```python
from build123d import *

# Parameters (mm, degrees)
SKETCH1_W                      = 15
SKETCH1_H                      = 1.65
SKETCH2_R                      = 6.95
BOSS_EXTRUDE1_DEPTH            = 10.8
F_5_0_5_DIAMETER_HOLE1_D       = 5
F_5_0_5_DIAMETER_HOLE1_DEPTH   = 12.45
F_3_0_3_DIAMETER_HOLE1_D       = 3
F_3_0_3_DIAMETER_HOLE1_DEPTH   = 12.45
F_9_8_9_8_DIAMETER_HOLE1_D     = 9.8
F_9_8_9_8_DIAMETER_HOLE1_DEPTH = 12.45
FILLET1_R                      = 0.5


with BuildPart() as part:
    # Sketch1 → Revolve1 (revolve)
    with BuildSketch(Plane(origin=(0, 0, 0), x_dir=(1, 0, 0), z_dir=(0, 1, 0))):
        with Locations((7.5, -0.825)):
            Rectangle(SKETCH1_W, SKETCH1_H)
    revolve(axis=Axis((0, 0, 0), (0, 0, 1)))

    # Sketch2 → Boss-Extrude1 (add)
    with BuildSketch(Plane.XY.offset(1.65)):
        Circle(SKETCH2_R)
    extrude(amount=BOSS_EXTRUDE1_DEPTH)

    # Ø5.0 (5) Diameter Hole1
    with Locations(Plane(origin=(0, 0, 0), x_dir=(-1, 0, 0), z_dir=(0, 0, -1))):
        with Locations((7.552754414, 9.001022207), (11.571491098, 2.040366088), (4.018736684, -11.041388294), (-4.018736684, -11.041388294), (-11.571491098, 2.040366088), (-7.552754414, 9.001022207)):
            Hole(F_5_0_5_DIAMETER_HOLE1_D / 2, depth=F_5_0_5_DIAMETER_HOLE1_DEPTH)

    # Ø3.0 (3) Diameter Hole1
    with Locations(Plane(origin=(0, 0, 0), x_dir=(-1, 0, 0), z_dir=(0, 0, -1))):
        with Locations((0, 11.75), (10.175798494, -5.875), (-10.175798494, -5.875)):
            Hole(F_3_0_3_DIAMETER_HOLE1_D / 2, depth=F_3_0_3_DIAMETER_HOLE1_DEPTH)

    # Ø9.8 (9.8) Diameter Hole1
    with Locations(Plane(origin=(0, 0, 0), x_dir=(-1, 0, 0), z_dir=(0, 0, -1))):
        with Locations((0, 0)):
            Hole(F_9_8_9_8_DIAMETER_HOLE1_D / 2, depth=F_9_8_9_8_DIAMETER_HOLE1_DEPTH)

    # Fillet1
    fillet1_edges = [part.edges().sort_by_distance(p)[0] for p in [
        (-4.9, 0, 0),
    ]]
    fillet(fillet1_edges, radius=FILLET1_R)


solid = part.part
```
Geometry check sheet. Reference: the model listing, model coordinates, mm. A direction names the side the tool comes from. Round coordinates to 2 decimals unless told otherwise and drop trailing zeros. Loops run counter-clockwise (first coordinate to the right, second up) from the corner with the lowest first, then second, coordinate; pieces in that order, holes last. Notation, with made-up numbers: M -18,48 L 38,48 A24 cw 38,86 Z; hole C 49.5,-3.5 d4. An arc over 180 degrees is marked long. Return JSON: item names as keys, results as strings. Group by question number.
(1) Section check B-B, the plane y = -11.75. Enter the section's corners in (x, z), and give its area (3 significant figures).
(2) Scan lines: line 1 along X through (y, z) = (-3.75, 8.5); line 2 along Z through (x, y) = (7.25, -9.25); line 3 along Y through (x, z) = (-2.5, 11.5). Record each from-to range of solid material in increasing order. Write a range as [from, to].
(3) Go/stop test with flat-tipped pins: pin 1 (3 mm diameter, centred on x = 10.5, y = -7, fed in from +Z); pin 2 (6 mm diameter, centred on x = 5.5, z = 8, fed in from -Y); pin 3 (1 mm diameter, centred on x = 5, z = 8, fed in from -Y). Record where each tip stops, or that it passes through.
(4) Mould release check, pull along Y, two halves, no side actions. Record for faces 3 (the face through (1, 5, 12.45)), 4 (the face through (-6.399, 6.783, 0.837)), 5 (the face through (-1.507, -6.785, 6.974)): pulls with the +Y half, pulls with the -Y half, needs draft (parallel to the pull), parting line crosses it, or undercut.
(5) Section check C-C, the plane z = 3.25. Enter the section's corners in (x, y).
(6) Section check A-A, the plane x = 0. Enter the section's corners in (y, z).
(7) Set-up check for faces 1 (the face through (-6.5, -3.1, 1.65)), 2 (the face through (7.01, 6.56, 0.84)): record each of +Z, -Z, +X, -X, +Y, -Y from which the full face is reachable in a straight line by a thin tool's end or side.
(8) Section check D-D, the plane y = 3.75. Give the number of separate pieces and of enclosed holes in the cut face, and give its area (3 significant figures).
Data:
{
 "1": {"outline": "M -9.32,0 L -6.42,0 L -6.42,1.65 L -9.32,1.65 Z; M -1.62,0 L 1.62,0 L 1.62,1.65 L -1.62,1.65 Z; M 6.42,0 L 9.32,0 L 9.32,1.65 L 6.42,1.65 Z", "area": "14.9 mm²"},
 "2": {"line 1": "[-5.85, -3.15], [3.15, 5.85]", "line 2": "[0, 1.65]", "line 3": "[-6.48, -4.21], [4.21, 6.48]"},
 "3": {"pin 1": "z = 1.65", "pin 2": "y = -6.48", "pin 3": "y = -5.3"},
 "4": {"face 3": "needs draft", "face 4": "undercut", "face 5": "parting line crosses it"},
 "5": {"outline": "C 0,0 d13.9; hole C 0,0 d9.8"},
 "6": {"outline": "M -15,0 L -5.4,0 A0.5 ccw -4.9,0.5 L -4.9,12.45 L -6.95,12.45 L -6.95,1.65 L -15,1.65 Z; M 4.9,0.5 A0.5 ccw 5.4,0 L 10.25,0 L 10.25,1.65 L 6.95,1.65 L 6.95,12.45 L 4.9,12.45 Z; M 13.25,0 L 15,0 L 15,1.65 L 13.25,1.65 Z"},
 "7": {"face 1": "+Z", "face 2": "+Z, -Z"},
 "8": {"separate pieces": "4", "enclosed holes": "0", "area": "83.6 mm²"}
}
